Build history of the part. All positions in model axes, mm. A direction names the side the tool comes from. Give positions to 0.01 mm unless a question says otherwise; leave off trailing zeros. Write each loop counter-clockwise with the first axis right and the second up, starting at its lowest first coordinate (ties: lowest second). Pieces come first, ordered by that corner, then holes. Notation, with made-up numbers: M -23,44.25 L 35,44.25 A10 ccw 35,53.25 Z; hole C -20.75,34.5 d9. An arc over 180 degrees is marked long. Return JSON: item names as keys, results as strings. Group by question number.
Q1. Band-saw the part on B-B, the plane x = 3. Give the cut face in (y, z), then the cut area to 3 significant figures.
Q2. Wall check: probe 1 along Y at (x, z) = (-36, 33); probe 2 along Y at (x, z) = (37.4, 4.4). Give the ranges that are in metal, low to high.
Q3. Pull direction Y, two halves, no side cores. Call faces 4 (the flat face through (-1, -46, 45)), 5 (the flat face through (-36, 36, 4)), 6 (the flat face through (-42, -1, 5)), 7 (the flat face through (43, -1, 89)): +Y half, -Y half, draft (parallel to the pull), parting line (faces both ways), or undercut.
Q4. Flat gauge pins, fed straight in: pin 1 Ø12 at (x, y) = (-19, 27) entering from -Z; pin 2 Ø11 at (x, y) = (-34, 34) entering from -Z; pin 3 Ø3 at (y, z) = (12.5, 2) entering from +X. Where does each tip first touch, or does it go through?
Q5. Band-saw the part on A-A, the plane z = 46.5. Give the cut face in (x, y).
Q6. Tool access for faces 1 (the cylindrical face through (36.184, 36.285, 4.641)), 2 (the flat face through (-1, 44.5, 45)), 3 (the flat face through (-42, -42, 4)): list every direction of +Z, -Z, +X, -X, +Y, -Y with a clear straight run to the whole face (end or side of a thin tool).
from build123d import *

# Parameters (mm, degrees)
F0_W      = 92
F0_H      = 92
F1_DEPTH  = 92
F2_SIZE   = 6
F3_DEPTH  = 80
F4_W      = 89
F4_H      = 89
F5_DEPTH  = 89
F6_SIZE   = 6
F17_DEPTH = 3.5
F10_R     = 1.65
F11_DEPTH = 1.3
F12_SIZE  = 0.49999
F15_DEPTH = 1.5


# Not quite as in the source:
# - a fillet or chamfer is up to 0.001 mm smaller than in the source, because OpenCascade refuses the exact size


with BuildPart() as f1:
    # F0 (on Top) → F1 (new body)
    with BuildSketch(Plane.XY):
        Rectangle(F0_W, F0_H)
    extrude(amount=F1_DEPTH)

    # F2
    f2_edges = [f1.edges().sort_by_distance(p)[0] for p in [
        (0, -46, 92),
        (46, 0, 92),
        (46, -46, 46),
        (0, -46, 0),
        (-46, -46, 46),
        (46, 0, 0),
        (46, 46, 46),
        (0, 46, 92),
        (-46, 0, 92),
        (-46, 0, 0),
        (-46, 46, 46),
        (0, 46, 0),
    ]]
    chamfer(f2_edges, length=F2_SIZE)

    # F3 (cut): a face of the model
    f3_faces = [f1.faces().sort_by_distance(p)[0] for p in [
        (0, 0, 0),
    ]]
    extrude(f3_faces, amount=-F3_DEPTH, mode=Mode.SUBTRACT)


with BuildPart() as f5:
    # F4 (on Top) → F5 (new body)
    with BuildSketch(Plane.XY):
        Rectangle(F4_W, F4_H)
    extrude(amount=F5_DEPTH)

    # F6
    f6_edges = [f5.edges().sort_by_distance(p)[0] for p in [
        (-44.5, -44.5, 44.5),
        (0, -44.5, 89),
        (44.5, -44.5, 44.5),
        (0, -44.5, 0),
        (44.5, 0, 89),
        (44.5, 44.5, 44.5),
        (44.5, 0, 0),
        (0, 44.5, 0),
        (-44.5, 0, 89),
        (0, 44.5, 89),
        (-44.5, 44.5, 44.5),
        (-44.5, 0, 0),
    ]]
    chamfer(f6_edges, length=F6_SIZE)


with BuildPart() as f5_1:
    # F7: moved
    add(f5.part.moved(Location((0, 0, 1.5))))


with BuildPart() as f1_1:
    add(f1.part)

    # F8: cut F5
    add(f5_1.part, mode=Mode.SUBTRACT)

    # F16 (on offset) → F17 (join)
    with BuildSketch(Plane.XY.offset(7.5)):
        Polygon((44.5, 26.0656665673), (44.5, 38.5), (38.5, 44.5), (26.0656665673, 44.5), (30.5656665673, 40), (40.5656665673, 30), align=None)
        Polygon((-25.5, 44.5), (-38.5, 44.5), (-44.5, 38.5), (-44.5, 25.5), (-40, 30), (-30, 40), align=None)
        Polygon((25.5, -44.5), (38.5, -44.5), (44.5, -38.5), (44.5, -25.5), (40, -30), (30, -40), align=None)
        Polygon((-44.5, -38.5), (-38.5, -44.5), (-26.5405371355, -44.5), (-30, -41.0405371355), (-40, -31.0405371355), (-44.5, -26.5405371355), align=None)
    extrude(amount=-F17_DEPTH)

    # F10 (on face) → F11 (cut)
    with BuildSketch(Plane(origin=(0, 0, 4), x_dir=(1, 0, 0), z_dir=(0, 0, -1))):
        with Locations((37.4, 37.4)):
            Circle(F10_R)
        with Locations((-37.4, 37.4)):
            Circle(F10_R)
        with Locations((-37.4, -37.4)):
            Circle(F10_R)
        with Locations((37.4, -37.4)):
            Circle(F10_R)
    extrude(amount=-F11_DEPTH, mode=Mode.SUBTRACT)

    # F12 (size 0.5 in the source; OpenCascade refuses exactly that, so slightly less here)
    f12_edges = [f1_1.edges().sort_by_distance(p)[0] for p in [
        (-32, 44.5, 4),
        (-44.5, 32, 4),
        (32.282833, 44.5, 4),
        (44.5, 32.282833, 4),
        (44.5, -32, 4),
        (-32.520269, -44.5, 4),
        (-44.5, -32.520269, 4),
        (32, -44.5, 4),
    ]]
    chamfer(f12_edges, length=F12_SIZE)

    # F14 (on face) → F15 (join)
    with BuildSketch(Plane(origin=(0, 0, 3), x_dir=(1, 0, 0), z_dir=(0, 0, -1))):
        Polygon((-41, 38.5), (-41, 30.0405371355), (-40, 31.0405371355), (-40, 39.5), (-40, 40), (-39.5, 40), (-31.0405371355, 40), (-30.0405371355, 41), (-38.5, 41), (-40, 41), (-41, 40), align=None)
        Polygon((38.5, 41), (29, 41), (30, 40), (39.5, 40), (40, 40), (40, 39.5), (40, 30), (41, 29), (41, 38.5), (41, 40), (40, 41), align=None)
        Polygon((41, -38.5), (41, -29.5656665673), (40, -30.5656665673), (40, -40), (30.5656665673, -40), (29.5656665673, -41), (38.5, -41), (40, -41), (41, -40), align=None)
        Polygon((-38.5, -41), (-29, -41), (-30, -40), (-40, -40), (-40, -30), (-41, -29), (-41, -38.5), (-41, -40), (-40, -41), align=None)
    extrude(amount=-F15_DEPTH)


solid = f1_1.part
From the geometry:
{
 "1": {"outline": "M -46,6 L -40,0 L -40,3 L -44.5,7.5 L -44.5,84.5 L -38.5,90.5 L 38.5,90.5 L 44.5,84.5 L 44.5,7.5 L 40,3 L 40,0 L 46,6 L 46,86 L 40,92 L -40,92 L -46,86 Z", "area": "421 mm^2"},
 "2": {"probe 1": "y = -46 to -44.5, 44.5 to 46", "probe 2": "y = -44.4 to -39.05, -35.75 to -32.6, 33.17 to 35.75, 39.05 to 44.4"},
 "3": {"face 4": "-Y half", "face 5": "undercut", "face 6": "undercut", "face 7": "draft"},
 "4": {"pin 1": "stops at z = 90.5", "pin 2": "stops at z = 4", "pin 3": "stops at x = 43.5"},
 "5": {"outline": "M -46,-40 L -40,-46 L 40,-46 L 46,-40 L 46,40 L 40,46 L -40,46 L -46,40 Z; hole M -44.5,-38.5 L -38.5,-44.5 L 38.5,-44.5 L 44.5,-38.5 L 44.5,38.5 L 38.5,44.5 L -38.5,44.5 L -44.5,38.5 Z"},
 "6": {"face 1": "-Z", "face 2": "none", "face 3": "-Z, -X, -Y"}
}
